Input: part model. Units: mm. Frame: model coordinates. Face numbers are marked on the shaded views. A direction names the side the tool comes from. Round coordinates to 2 decimals unless told otherwise and drop trailing zeros. Order: outer loops, then holes, each group sorted by start corner. A loop starts at its lowest first (then second) coordinate and runs counter-clockwise, first axis right, second up. Notation, with made-up numbers: M 34.25,-32.75 L 80.25,-32.75 A27 cw 80.25,3.25 Z; hole C 15.5,5 d9. An arc over 180 degrees is marked long. One line per question, with ' | ' between items.
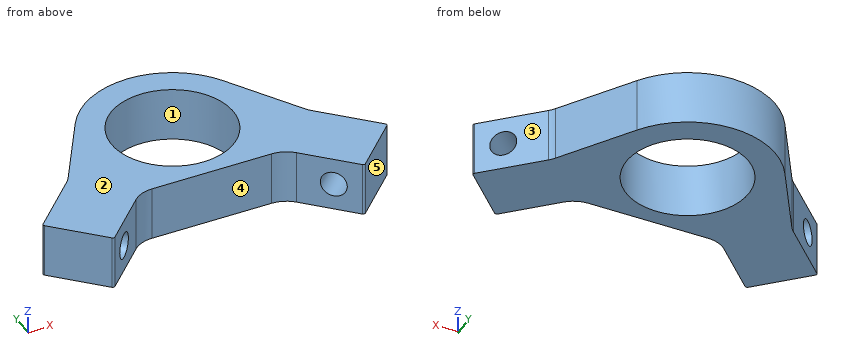
```python
from build123d import *

# Parameters (mm, degrees)
BOSS_EXTRUDE1_DEPTH             = 6.35
SKETCH2_R                       = 14.2875
CUT_EXTRUDE1_DEPTH              = 141.169556232
F_6_0MM_CLEARANCE_DOWEL_HOLE1_D = 6
CUT_EXTRUDE2_DEPTH              = 77.016140262
CUT_EXTRUDE3_DEPTH              = 55.213982826
FILLET1_R                       = 6.858
FILLET2_R                       = 0.508


with BuildPart() as part:
    # Sketch1 → Boss-Extrude1 (new, symmetric)
    with BuildSketch(Plane.XY):
        Polygon((-48.967108015, -44.583045972), (-17.084062043, -12.7), (17.084062043, -12.7), (48.967108015, -44.583045972), (60.245461175, -33.304692812), (28.575, -1.634231637), (28.575, 33.007903412), (-28.575, 33.007903412), (-28.575, -1.634231637), (-60.245461175, -33.304692812), align=None)
    extrude(amount=BOSS_EXTRUDE1_DEPTH, both=True)

    # Sketch2 → Cut-Extrude1 (cut, through all)
    with BuildSketch(Plane(origin=(0, -92.915481637, 6.35), x_dir=(1, 0, 0), z_dir=(0, 0, 1))):
        with Locations((0, 98.425)):
            Circle(SKETCH2_R)
    extrude(amount=-CUT_EXTRUDE1_DEPTH, mode=Mode.SUBTRACT)

    # Ø6.0mm Clearance Dowel Hole1 (through all)
    with Locations(Plane(origin=(-59.928125, -32.987356637, 33.65), x_dir=(0, 0, 1), z_dir=(-0.7071067811865488, 0.7071067811865464, 0))):
        with Locations((-33.65, 33.499886537)):
            f_6_0mm_clearance_dowel_hole1 = Hole(F_6_0MM_CLEARANCE_DOWEL_HOLE1_D / 2)

    # Sketch5 → Cut-Extrude2 (cut, through all)
    with BuildSketch(Plane.XY.offset(6.35)):
        Polygon((-41.089466366, -14.148698003), (-29.811113206, -25.427051163), (29.811113206, -25.427051163), (41.089466366, -14.148698003), (91.882290576, -14.148698003), (91.882290576, -80.233341252), (-80.675634817, -80.233341252), (-80.675634817, -14.148698003), align=None)
    extrude(amount=-CUT_EXTRUDE2_DEPTH, mode=Mode.SUBTRACT)

    # Mirror1: Ø6.0mm Clearance Dowel Hole1 across plane
    add(f_6_0mm_clearance_dowel_hole1.mirror(Plane(origin=(0, 0, 0), x_dir=(0, 0, 1), z_dir=(1, 0, 0))), mode=Mode.SUBTRACT)

    # Sketch6 → Cut-Extrude3 (cut, through all)
    with BuildSketch(Plane.XY.offset(6.35)):
        with BuildLine():
            Line((-28.575, -1.634231637), (-17.599390848, 16.28763731))
            ThreePointArc((-17.599390848, 16.28763731), (0, 26.147018363), (17.599390848, 16.28763731))
            Line((17.599390848, 16.28763731), (28.575, -1.634231637))
            Line((28.575, -1.634231637), (28.575, 33.007903412))
            Line((28.575, 33.007903412), (-28.575, 33.007903412))
            Line((-28.575, 33.007903412), (-28.575, -1.634231637))
        make_face()
    extrude(amount=-CUT_EXTRUDE3_DEPTH, mode=Mode.SUBTRACT)

    # Fillet1
    fillet1_edges = [part.edges().sort_by_distance(p)[0] for p in [
        (-28.575, -1.634231637, 0),
        (28.575, -1.634231637, 0),
        (17.084062043, -12.7, 0),
        (-17.084062043, -12.7, 0),
    ]]
    fillet(fillet1_edges, radius=FILLET1_R)

    # Fillet2
    fillet2_edges = [part.edges().sort_by_distance(p)[0] for p in [
        (-41.089466366, -14.148698003, 0),
        (-29.811113206, -25.427051163, 0),
        (29.811113206, -25.427051163, 0),
        (41.089466366, -14.148698003, 0),
    ]]
    fillet(fillet2_edges, radius=FILLET2_R)


solid = part.part
```
Item 1: First-contact query: pin 1 (3 mm diameter, centred on y = -9, z = -0.5, fed in from -X); pin 2 (4 mm diameter, centred on x = 0, z = -2, fed in from -Y); pin 3 (17 mm diameter, centred on x = 0, y = 5.51, fed in from -Z); pin 4 (2 mm diameter, centred on y = 13, z = -4.5, fed in from -X). Flat tips, straight axial feed; report the tip coordinate or a pass-through.
Report:
pin 1: x = -33.99 | pin 2: y = -12.7 | pin 3: through | pin 4: x = -20.23
Item 2: Mould query, pull axis Y, two halves, no side actions, for the marked faces 1, 2 and 3. Classes: +Y half, -Y half, draft (parallel to the pull), parting line (faces both ways), or undercut.
Report:
face 1: undercut | face 2: draft | face 3: +Y half
Item 3: Access query for the marked faces 4 and 5. Directions: +Z, -Z, +X, -X, +Y, -Y. A direction counts if a zero-diameter tool reaches every point of the face in a straight line with its end or side. Return the directions, or none.
Report:
face 4: +Z, -Z, -Y | face 5: +Z, -Z, +X, -Y
Item 4: Line query: line 1 along Y through (x, z) = (0, -3.5); line 2 along X through (y, z) = (-20, 0.75); line 3 along Y through (x, z) = (12, -2.75) (3 decimals). Output: solid intervals per line, ascending. Write a range as from..to.
Report:
line 1: -12.7..-8.78, 19.8..26.15 | line 2: -35.24..-29.65, 29.65..35.24 | line 3: -12.7..-2.245, 13.264..22.3
Item 5: Section query C-C, the plane y = 1. Return loops of the section in (x, z), plus the area to 3 significant figures.
Report:
outline: M -26.96,-6.35 L -13.56,-6.35 L -13.56,6.35 L -26.96,6.35 Z; M 13.56,-6.35 L 26.96,-6.35 L 26.96,6.35 L 13.56,6.35 Z | area: 340 mm²
Item 6: Section query B-B, the plane x = 0. Return loops of the section in (y, z).
Report:
outline: M -12.7,-6.35 L -8.78,-6.35 L -8.78,6.35 L -12.7,6.35 Z; M 19.8,-6.35 L 26.15,-6.35 L 26.15,6.35 L 19.8,6.35 Z
Item 7: Section query A-A, the plane z = 1.5. Return loops of the section in (x, y) (1 decimal).
Report:
outline: M -40.7,-14.5 L -30.2,-25.1 A0.5 ccw -29.5,-25.1 L -26.8,-22.4 L -38.1,-11.1 L -40.7,-13.8 A0.5 ccw Z; M -34.4,-7.5 L -23.1,-18.7 L -19.1,-14.7 A6.9 cw -14.2,-12.7 L 14.2,-12.7 A6.9 cw 19.1,-14.7 L 23.1,-18.7 L 34.4,-7.5 L 29.1,-2.2 A6.9 cw 28.2,-0.9 L 17.6,16.3 A20.6 ccw -17.6,16.3 L -28.2,-0.9 A6.9 cw -29.1,-2.2 Z; M 26.8,-22.4 L 29.5,-25.1 A0.5 ccw 30.2,-25.1 L 40.7,-14.5 A0.5 ccw 40.7,-13.8 L 38.1,-11.1 Z; hole C 0,5.5 d28.6
